Geometry check sheet. Reference: the model listing, model coordinates, mm. Round coordinates to 2 decimals unless told otherwise and drop trailing zeros. Write each loop counter-clockwise with the first axis right and the second up, starting at its lowest first coordinate (ties: lowest second). Pieces come first, ordered by that corner, then holes. Notation, with made-up numbers: M 9.25,2 L 45.25,2 A38 cw 45.25,40 Z; hole C 12.25,29 d9. An arc over 180 degrees is marked long. Answer in a Markdown table with one row per item. Add a question column.
from build123d import *

# Parameters (mm, degrees)
FILLET1_R          = 0.3
CUT_EXTRUDE1_DEPTH = 0.88


with BuildPart() as part:
    # Sketch1 → Revolve1 (revolve)
    with BuildSketch(Plane.XY, mode=Mode.PRIVATE) as revolve1_sk:
        Polygon((-1.75, 0), (-1.75, 3), (-1.5, 3), (0.155, 1.345), (1.005, 1.345), (1.005, 1.5), (3.25, 1.5), (3.25, 0), align=None)
    revolve(revolve1_sk.sketch.rotate(Axis((-1.75, 0, 0), (1, 0, 0)), 180), axis=Axis((-1.75, 0, 0), (1, 0, 0)))

    # Fillet1
    fillet1_edges = [part.edges().sort_by_distance(p)[0] for p in [
        (0.155, 1.345, 0),
    ]]
    fillet(fillet1_edges, radius=FILLET1_R)

    # Sketch2 → Cut-Extrude1 (cut)
    with BuildSketch(Plane.ZY.offset(1.75)):
        with BuildLine():
            Line((-0.4, 1.8), (0.4, 1.8))
            Line((0.4, 1.8), (0.4, 1))
            ThreePointArc((0.4, 1), (0.575735931, 0.575735931), (1, 0.4))
            Line((1, 0.4), (1.8, 0.4))
            Line((1.8, 0.4), (1.8, -0.4))
            Line((1.8, -0.4), (1, -0.4))
            ThreePointArc((1, -0.4), (0.575735931, -0.575735931), (0.4, -1))
            Line((0.4, -1), (0.4, -1.8))
            Line((0.4, -1.8), (-0.4, -1.8))
            Line((-0.4, -1.8), (-0.4, -1))
            ThreePointArc((-0.4, -1), (-0.575735931, -0.575735931), (-1, -0.4))
            Line((-1, -0.4), (-1.8, -0.4))
            Line((-1.8, -0.4), (-1.8, 0.4))
            Line((-1.8, 0.4), (-1, 0.4))
            ThreePointArc((-1, 0.4), (-0.575735931, 0.575735931), (-0.4, 1))
            Line((-0.4, 1), (-0.4, 1.8))
        make_face()
    extrude(amount=-CUT_EXTRUDE1_DEPTH, mode=Mode.SUBTRACT)


solid = part.part
Item 1: Section check B-B, the plane x = 2.75. Record the boundary of the cut face in (y, z), and give its area (3 significant figures).
Item 2: Section check A-A, the plane x = -0.95. Record the boundary of the cut face in (y, z), and give its area (3 significant figures).
Item 3: Scan lines: probe 1 along X at (y, z) = (0.25, -0.25); probe 2 along Z at (x, y) = (-1.25, -1.5); probe 3 along Y at (x, z) = (-1.2, -1). Record each from-to range of solid material in increasing order. Write a range as from..to.
Item 4: Mould release check, pull along X, two halves, no side actions. Record for faces 1 (the cylindrical face through (2.14, -1.43, -0.45)), 2 (the cylindrical face through (0.65, -1.24, 0.52)), 3 (the flat face through (-0.87, 0, 0)): +X half, -X half, draft (parallel to the pull), parting line (faces both ways), or undercut.
Item 5: Section check C-C, the plane x = 0.6. Record the boundary of the cut face in (y, z) (3 decimals).
Item 6: Gauge pin test, flat ends, axial feed: pin 1 Ø0.6 at (x, z) = (-1, -1) entering from -Y; pin 2 Ø1.5 at (x, y) = (0.5, 0.5) entering from +Z; pin 3 Ø1.5 at (x, z) = (2, 1) entering from +Y. Record the tip position at first contact, or that the pin passes through.
Result sheet:
| question | item | result |
|---|---|---|
| 1 | outline | C 0,0 d3 |
| 1 | area | 7.07 mm^2 |
| 2 | outline | C 0,0 d4.9; hole M -1.8,-0.4 L -1,-0.4 A0.6 cw -0.4,-1 L -0.4,-1.8 L 0.4,-1.8 L 0.4,-1 A0.6 cw 1,-0.4 L 1.8,-0.4 L 1.8,0.4 L 1,0.4 A0.6 cw 0.4,1 L 0.4,1.8 L -0.4,1.8 L -0.4,1 A0.6 cw -1,0.4 L -1.8,0.4 Z |
| 2 | area | 13.4 mm^2 |
| 3 | probe 1 | x = -0.87..3.25 |
| 3 | probe 2 | z = -2.3..-0.4, 0.4..2.3 |
| 3 | probe 3 | y = -2.51..-0.4, 0.4..2.51 |
| 4 | face 1 | draft |
| 4 | face 2 | undercut |
| 4 | face 3 | -X half |
| 5 | outline | C 0,0 d2.69 |
| 6 | pin 1 | stops at y = -2.63 |
| 6 | pin 2 | stops at z = 1.7 |
| 6 | pin 3 | stops at y = 1.48 |
